from build123d import *

# Parameters (mm, degrees)
CHAMFER1_SIZE = 2.1


with BuildPart() as part:
    # Sketch1 → Revolve1 (revolve)
    with BuildSketch(Plane.XY, mode=Mode.PRIVATE) as revolve1_sk:
        with BuildLine():
            Line((-15.170481252, 65), (15.829518748, 65))
            Line((15.829518748, 65), (15.829518748, 53))
            Line((15.829518748, 53), (9.329518748, 53))
            ThreePointArc((9.329518748, 53), (0.329518748, 57.062746067), (-8.670481252, 53))
            Line((-8.670481252, 53), (-15.170481252, 53))
            Line((-15.170481252, 53), (-15.170481252, 65))
        make_face()
    revolve(revolve1_sk.sketch.rotate(Axis((-8.519406172, 0, 0), (1, 0, 0)), 90), axis=Axis((-8.519406172, 0, 0), (1, 0, 0)))

    # Chamfer1
    chamfer1_edges = [part.edges().sort_by_distance(p)[0] for p in [
        (15.829518748, 0, -65),
        (-15.170481252, 0, -65),
    ]]
    chamfer(chamfer1_edges, length=CHAMFER1_SIZE)


solid = part.part
Geometry check sheet. Reference: the model listing, model coordinates, mm. Give positions to 0.01 mm unless a question says otherwise; leave off trailing zeros. Write each loop counter-clockwise with the first axis right and the second up, starting at its lowest first coordinate (ties: lowest second). Pieces come first, ordered by that corner, then holes.
1) Go/stop test with flat-tipped pins: pin 1 Ø1.5 at (x, y) = (-10, 39.5) entering from -Z; pin 2 Ø3 at (x, z) = (0.5, -14.5) entering from -Y; pin 3 Ø3 at (x, y) = (1, 51) entering from -Z. Record where each tip stops, or that it passes through.
Values follow:
pin 1: stops at z = -52.19
pin 2: stops at y = -63.69
pin 3: stops at z = -42.13
2) Release check for a two-part mould opening along Y. For faces 1 (the face through (12.53, -52.55, -6.9)), 2 (the face through (-11.97, -52.55, -6.9)), 3 (the face through (15.83, 42, -33)), 4 (the face through (0.52, -19.52, 62)) record: released by +Y, released by -Y, zero draft, split by the parting line, or undercut.
Values follow:
face 1: undercut
face 2: undercut
face 3: zero draft
face 4: split by the parting line
3) Cross-section at A-A (z = 0). Record the boundary of the cut face in (x, y), plus the area to 3 significant figures.
Values follow:
outline: (-15.17, -62.9) - (-13.07, -65) - (13.73, -65) - (15.83, -62.9) - (15.83, -53) - (9.33, -53) arc R12 cw to (-8.67, -53) - (-15.17, -53) - close; (-15.17, 53) - (-8.67, 53) arc R12 cw to (9.33, 53) - (15.83, 53) - (15.83, 62.9) - (13.73, 65) - (-13.07, 65) - (-15.17, 62.9) - close
area: 634 mm2
4) Cross-section at D-D (x = 2). Record the boundary of the cut face in (y, z), plus the area to 3 significant figures.
Values follow:
outline: circle Ø130 at (0, 0); hole circle Ø113.89 at (0, 0)
area: 3,090 mm2
5) Thickness scan on line 1 (Y direction, x = 12, z = 0); line 2 (Y direction, x = -13.75, z = 0); line 3 (Z direction, x = -7.5, y = -47.5). Record the ranges inside material, lowest first.
Values follow:
line 1: y = -65 to -53, 53 to 65
line 2: y = -64.32 to -53, 53 to 64.32
line 3: z = -44.37 to -26.01, 26.01 to 44.37
6) Cross-section at C-C (x = -11). Record the boundary of the cut face in (y, z).
Values follow:
outline: circle Ø130 at (0, 0); hole circle Ø106 at (0, 0)
